Design review of the part built by this model. Coordinates are the model's own, in mm. Face numbers are marked on the shaded views. A direction names the side the tool comes from. Round coordinates to 2 decimals unless told otherwise and drop trailing zeros. Write each loop counter-clockwise with the first axis right and the second up, starting at its lowest first coordinate (ties: lowest second). Pieces come first, ordered by that corner, then holes. Notation, with made-up numbers: (-12, 4) - (-4, 4) arc R21 cw to (-4, 28) - close; hole circle Ø8 at (-37.5, -32). An arc over 180 degrees is marked (long way). Use one line per item in the form item = value.
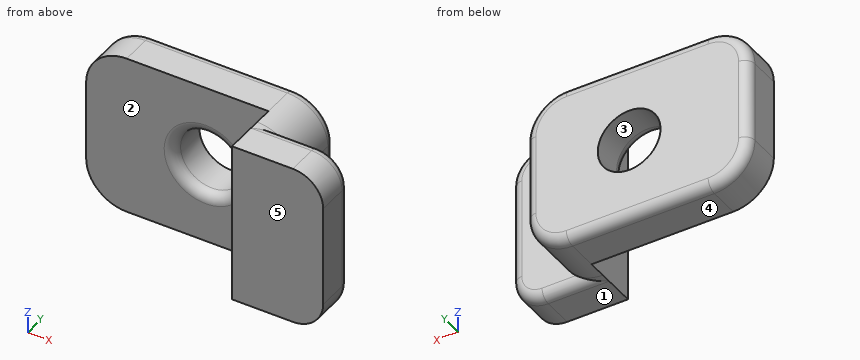
```python
from build123d import *

# Parameters (mm, degrees)
BOSS_EXTRUDE1_DEPTH     = 2
CUT_EXTRUDE1_DEPTH      = 8.088723439
CUT_EXTRUDE1_DEPTH_BACK = 8.088723439
SKETCH2_R               = 1.55
BOSS_EXTRUDE2_START     = 2.9
BOSS_EXTRUDE2_DEPTH     = 2.9
BOSS_EXTRUDE3_DEPTH     = 2
FILLET1_R               = 0.5


with BuildPart() as part:
    # Sketch1 → Boss-Extrude1 (new body)
    with BuildSketch(Plane(origin=(0, 0, 0), x_dir=(1, 0, 0), z_dir=(0, 1, 0))):
        with BuildLine():
            Line((3.5, 4), (-3.5, 4))
            ThreePointArc((-3.5, 4), (-4.914213562, 3.414213562), (-5.5, 2))
            Line((-5.5, 2), (-5.5, -2))
            ThreePointArc((-5.5, -2), (-4.914213562, -3.414213562), (-3.5, -4))
            Line((-3.5, -4), (3.5, -4))
            ThreePointArc((3.5, -4), (4.914213562, -3.414213562), (5.5, -2))
            Line((5.5, -2), (5.5, 2))
            ThreePointArc((5.5, 2), (4.914213562, 3.414213562), (3.5, 4))
        make_face()
    extrude(amount=BOSS_EXTRUDE1_DEPTH)

    # Sketch2 → Cut-Extrude1 (cut, two sides: drawn at the far end of the back side and taken through both)
    with BuildSketch(Plane(origin=(0, 2, 0), x_dir=(1, 0, 0), z_dir=(0, 1, 0)).offset(-CUT_EXTRUDE1_DEPTH_BACK)):
        with Locations(Location((0.4, 0, 0), (0, 0, 270))):
            Circle(SKETCH2_R)
    extrude(amount=CUT_EXTRUDE1_DEPTH + CUT_EXTRUDE1_DEPTH_BACK, mode=Mode.SUBTRACT)

    # Sketch3 → Boss-Extrude2 (add)
    with BuildSketch(Plane.XZ.offset(BOSS_EXTRUDE2_START)):
        with BuildLine():
            Line((5.5, 2), (5.5, -2))
            ThreePointArc((5.5, -2), (4.914213562, -3.414213562), (3.5, -4))
            Line((3.5, -4), (3.5, 4))
            ThreePointArc((3.5, 4), (4.914213562, 3.414213562), (5.5, 2))
        make_face()
    extrude(amount=-BOSS_EXTRUDE2_DEPTH)

    # Sketch4 → Boss-Extrude3 (add)
    with BuildSketch(Plane.XZ.offset(2.9)):
        with BuildLine():
            Line((5.5, 2), (5.5, -2))
            ThreePointArc((5.5, -2), (4.914213562, -3.414213562), (3.5, -4))
            Line((3.5, -4), (6.5, -4))
            ThreePointArc((6.5, -4), (7.560660172, -3.560660172), (8, -2.5))
            Line((8, -2.5), (8, 2.5))
            ThreePointArc((8, 2.5), (7.560660172, 3.560660172), (6.5, 4))
            Line((6.5, 4), (3.5, 4))
            ThreePointArc((3.5, 4), (4.914213562, 3.414213562), (5.5, 2))
        make_face()
    extrude(amount=-BOSS_EXTRUDE3_DEPTH)

    # Fillet1
    # the kernel refuses this fillet: 0.5 mm, written as the material it takes off along each edge
    with BuildSketch(Plane(origin=(-3.5, 2, 2), x_dir=(-1, 0, 0), z_dir=(0, 0, -1))) as fillet1_piece_1:
        with BuildLine():
            CenterArc((2 - FILLET1_R, -FILLET1_R), FILLET1_R, 0, 90)
            Line((2, -FILLET1_R), (2, 0))
            Line((2, 0), (2 - FILLET1_R, 0))
        make_face()
    revolve(axis=Axis((-3.5, 2, 2), (0, 1, 0)), revolution_arc=90, mode=Mode.SUBTRACT)
    with BuildSketch(Plane(origin=(-3.5, 2, 4), x_dir=(0, 0, -1), z_dir=(1, 0, 0)), Plane(origin=(3.5, 2, -4), x_dir=(0, 0, 1), z_dir=(-1, 0, 0))) as fillet1_piece_2:
        with BuildLine():
            CenterArc((FILLET1_R, -FILLET1_R), FILLET1_R, 90, 90)
            Line((0, -FILLET1_R), (0, 0))
            Line((0, 0), (FILLET1_R, 0))
        make_face()
    extrude(amount=7, mode=Mode.SUBTRACT)
    with BuildSketch(Plane(origin=(3.5, 2, 2), x_dir=(0, 0, 1), z_dir=(-1, 0, 0))) as fillet1_piece_3:
        with BuildLine():
            CenterArc((2 - FILLET1_R, -FILLET1_R), FILLET1_R, 0, 90)
            Line((2 - FILLET1_R, 0), (2, 0))
            Line((2, 0), (2, -FILLET1_R))
        make_face()
    revolve(axis=Axis((3.5, 2, 2), (0, 1, 0)), revolution_arc=90, mode=Mode.SUBTRACT)
    with BuildSketch(Plane(origin=(5.5, 2, 2), x_dir=(0, -1, 0), z_dir=(0, 0, -1))) as fillet1_piece_4:
        with BuildLine():
            CenterArc((FILLET1_R, FILLET1_R), FILLET1_R, 180, 90)
            Line((0, FILLET1_R), (0, 0))
            Line((0, 0), (FILLET1_R, 0))
        make_face()
    extrude(amount=4, mode=Mode.SUBTRACT)
    with BuildSketch(Plane(origin=(0.4, 0, 0), x_dir=(0, 0, 1), z_dir=(-1, 0, 0))) as fillet1_piece_5:
        with BuildLine():
            CenterArc((1.55 + FILLET1_R, FILLET1_R), FILLET1_R, 180, 90)
            Line((1.55 + FILLET1_R, 0), (1.55, 0))
            Line((1.55, 0), (1.55, FILLET1_R))
        make_face()
    revolve(axis=Axis((0.4, 0, 0), (0, 1, 0)), mode=Mode.SUBTRACT)
    with BuildSketch(Plane(origin=(3.5, 2, -2), x_dir=(1, 0, 0), z_dir=(0, 0, 1))) as fillet1_piece_6:
        with BuildLine():
            CenterArc((2 - FILLET1_R, -FILLET1_R), FILLET1_R, 0, 90)
            Line((2 - FILLET1_R, 0), (2, 0))
            Line((2, 0), (2, -FILLET1_R))
        make_face()
    revolve(axis=Axis((3.5, 2, -2), (0, 1, 0)), revolution_arc=90, mode=Mode.SUBTRACT)
    with BuildSketch(Plane(origin=(6.5, -0.9, 4), x_dir=(0, 0, -1), z_dir=(-1, 0, 0))) as fillet1_piece_7_section:
        with BuildLine():
            CenterArc((FILLET1_R, FILLET1_R), FILLET1_R, 180, 90)
            Line((0, FILLET1_R), (0, 0))
            Line((0, 0), (FILLET1_R, 0))
        make_face()
    fillet1_piece_7 = extrude(amount=4.25, mode=Mode.PRIVATE)
    fillet1_piece_7 = fillet1_piece_7 - Plane(origin=(3.5, -0.984531393, 2), x_dir=(0, 0, 1), z_dir=(0, -1, 0)) * Cylinder(2, 11, mode=Mode.PRIVATE)
    add(fillet1_piece_7, mode=Mode.SUBTRACT)
    with BuildSketch(Plane(origin=(6.5, -0.9, 2.5), x_dir=(1, 0, 0), z_dir=(0, 0, -1))) as fillet1_piece_8:
        with BuildLine():
            CenterArc((1.5 - FILLET1_R, FILLET1_R), FILLET1_R, 270, 90)
            Line((1.5, FILLET1_R), (1.5, 0))
            Line((1.5, 0), (1.5 - FILLET1_R, 0))
        make_face()
    revolve(axis=Axis((6.5, -0.9, 2.5), (0, -1, 0)), revolution_arc=90, mode=Mode.SUBTRACT)
    with BuildSketch(Plane(origin=(8, -0.9, -2.5), x_dir=(-1, 0, 0), z_dir=(0, 0, 1))) as fillet1_piece_9:
        with BuildLine():
            CenterArc((FILLET1_R, FILLET1_R), FILLET1_R, 180, 90)
            Line((0, FILLET1_R), (0, 0))
            Line((0, 0), (FILLET1_R, 0))
        make_face()
    extrude(amount=5, mode=Mode.SUBTRACT)
    with BuildSketch(Plane(origin=(6.5, -0.9, -2.5), x_dir=(0, 0, -1), z_dir=(-1, 0, 0))) as fillet1_piece_10:
        with BuildLine():
            CenterArc((1.5 - FILLET1_R, FILLET1_R), FILLET1_R, 270, 90)
            Line((1.5, FILLET1_R), (1.5, 0))
            Line((1.5, 0), (1.5 - FILLET1_R, 0))
        make_face()
    revolve(axis=Axis((6.5, -0.9, -2.5), (0, -1, 0)), revolution_arc=90, mode=Mode.SUBTRACT)
    with BuildSketch(Plane(origin=(2.25, -0.9, -4), x_dir=(0, 0, 1), z_dir=(1, 0, 0))) as fillet1_piece_11_section:
        with BuildLine():
            CenterArc((FILLET1_R, FILLET1_R), FILLET1_R, 180, 90)
            Line((0, FILLET1_R), (0, 0))
            Line((0, 0), (FILLET1_R, 0))
        make_face()
    fillet1_piece_11 = extrude(amount=4.25, mode=Mode.PRIVATE)
    fillet1_piece_11 = fillet1_piece_11 - Plane(origin=(3.5, -1.027464109, -2), x_dir=(1, 0, 0), z_dir=(0, -1, 0)) * Cylinder(2, 11, mode=Mode.PRIVATE)
    add(fillet1_piece_11, mode=Mode.SUBTRACT)
    with BuildSketch(Plane(origin=(-3.5, 2, -2), x_dir=(0, 0, -1), z_dir=(1, 0, 0))) as fillet1_piece_12:
        with BuildLine():
            CenterArc((2 - FILLET1_R, -FILLET1_R), FILLET1_R, 0, 90)
            Line((2, -FILLET1_R), (2, 0))
            Line((2, 0), (2 - FILLET1_R, 0))
        make_face()
    revolve(axis=Axis((-3.5, 2, -2), (0, 1, 0)), revolution_arc=90, mode=Mode.SUBTRACT)
    with BuildSketch(Plane(origin=(-5.5, 2, -2), x_dir=(1, 0, 0), z_dir=(0, 0, 1))) as fillet1_piece_13:
        with BuildLine():
            CenterArc((FILLET1_R, -FILLET1_R), FILLET1_R, 90, 90)
            Line((0, -FILLET1_R), (0, 0))
            Line((0, 0), (FILLET1_R, 0))
        make_face()
    extrude(amount=4, mode=Mode.SUBTRACT)


solid = part.part
```
Q1. For P1, Ø3, axis at x = 0.4, z = 0, coming from the -Y side; P2, Ø2.5, axis at y = -2, z = 1.5, coming from the -X side; P3, Ø0.8, axis at x = 6.5, z = -1, coming from the +Y side; P4, Ø1.2, axis at y = 0.5, z = 0, coming from the +X side, all flat-tipped, find the tip position at first contact; note any pin that passes through.
Calculated:
P1 = through
P2 = 3.5
P3 = -0.9
P4 = 5.5
Q2. Draft analysis for pull direction Z (two halves, no side actions). For the marked faces 3, 4 and 5, state which applies: released by +Z, released by -Z, zero draft, split by the parting line, or undercut.
Calculated:
face_3 = undercut
face_4 = released by -Z
face_5 = zero draft
Q3. We need section D-D on y = -2.05. Write out the cut boundary in (x, z).
Calculated:
outline = (3.5, -4) - (6.5, -4) arc R1.5 ccw to (8, -2.5) - (8, 2.5) arc R1.5 ccw to (6.5, 4) - (3.5, 4) - close
Q4. We need section B-B on x = 0.4. Write out the cut boundary in (y, z).
Calculated:
outline = (0, -4) - (1.5, -4) arc R0.5 ccw to (2, -3.5) - (2, -1.55) - (0.5, -1.55) arc R0.5 ccw to (0, -2.05) - close; (0, 2.05) arc R0.5 ccw to (0.5, 1.55) - (2, 1.55) - (2, 3.5) arc R0.5 ccw to (1.5, 4) - (0, 4) - close
Q5. We need section C-C on y = 0.9. Write out the cut boundary in (x, z).
Calculated:
outline = (-5.5, -2) arc R2 ccw to (-3.5, -4) - (3.5, -4) arc R2 ccw to (5.5, -2) - (5.5, 2) arc R2 ccw to (3.5, 4) - (-3.5, 4) arc R2 ccw to (-5.5, 2) - close; hole circle Ø3.1 at (0.4, 0)
Q6. To check wall thickness, follow line 1 along Z through (x, y) = (0.4, 1.3); line 2 along X through (y, z) = (1.3, 0); line 3 along Y through (x, z) = (5.75, -2.75). State the ranges of each line that lie inside material, in increasing order. Write a range as from..to.
Calculated:
line_1 = -4..-1.55, 1.55..4
line_2 = -5.5..-1.15, 1.95..5.5
line_3 = -2.9..-0.9
Q7. We need section A-A on z = 0. Write out the cut boundary in (x, y).
Calculated:
outline = (-5.5, 0) - (-1.65, 0) arc R0.5 ccw to (-1.15, 0.5) - (-1.15, 2) - (-5, 2) arc R0.5 ccw to (-5.5, 1.5) - close; (1.95, 0.5) arc R0.5 ccw to (2.45, 0) - (3.5, 0) - (3.5, -2.9) - (8, -2.9) - (8, -1.4) arc R0.5 ccw to (7.5, -0.9) - (5.5, -0.9) - (5.5, 1.5) arc R0.5 ccw to (5, 2) - (1.95, 2) - close
Q8. Machinability: for the marked faces 1 and 2, which of the approach directions +Z, -Z, +X, -X, +Y, -Y give a long, thin tool a straight path to every point of the face, cutting with its end or side? Answer none if there is none.
Calculated:
face_1 = -Z, +X, -X, +Y, -Y
face_2 = +Z, -Z, -X, -Y
